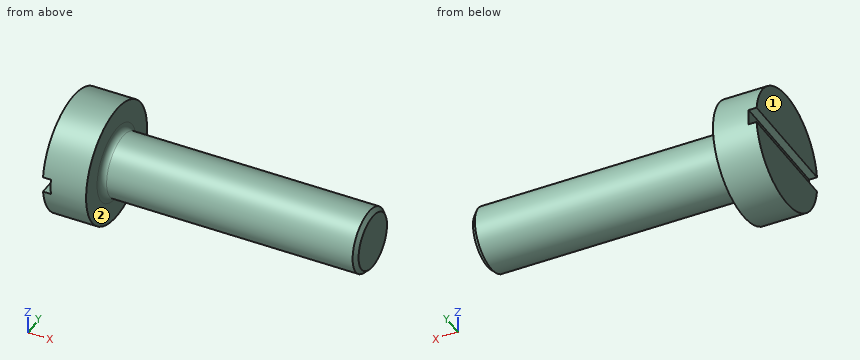
from build123d import *

# Parameters (mm, degrees)
SKETCH1_W           = 6.5
SKETCH1_H           = 0.8
CHAMFER1_SIZE       = 0.1
FILLET1_R           = 0.16
EXTRUDE1_DEPTH      = 8.890500618
EXTRUDE1_DEPTH_BACK = 8.890500618
SKETCH2_W           = 0.2
SKETCH2_H           = 0.2


with BuildPart() as part:
    # Sketch1 → Revolve1 (revolve)
    with BuildSketch(Plane.XY, mode=Mode.PRIVATE) as revolve1_sk:
        Polygon((0, 1.5), (0, 0), (1.1, 0), (1.1, 0.8), (1.1, 1.5), align=None)
        with Locations((4.35, 0.4)):
            Rectangle(SKETCH1_W, SKETCH1_H)
    revolve(revolve1_sk.sketch.rotate(Axis((0, 0, 0), (1, 0, 0)), 90), axis=Axis((0, 0, 0), (1, 0, 0)))

    # Chamfer1
    chamfer1_edges = [part.edges().sort_by_distance(p)[0] for p in [
        (7.6, 0, -0.8),
    ]]
    chamfer(chamfer1_edges, length=CHAMFER1_SIZE)

    # Fillet1
    fillet1_edges = [part.edges().sort_by_distance(p)[0] for p in [
        (1.1, 0, -0.8),
    ]]
    fillet(fillet1_edges, radius=FILLET1_R)

    # Sketch2 → Extrude1 (cut, two sides: drawn at the far end of the back side and taken through both)
    with BuildSketch(Plane(origin=(0, 0, 0), x_dir=(1, 0, 0), z_dir=(0, 1, 0)).offset(-EXTRUDE1_DEPTH_BACK)):
        with Locations((0.1, -0.1)):
            Rectangle(SKETCH2_W, SKETCH2_H)
        with Locations((0.1, 0.1)):
            Rectangle(SKETCH2_W, SKETCH2_H)
    extrude(amount=EXTRUDE1_DEPTH + EXTRUDE1_DEPTH_BACK, mode=Mode.SUBTRACT)


solid = part.part
Can you work these out from the model? Positions are in its coordinate system, mm. Face numbers are marked on the shaded views. A direction names the side the tool comes from. Coordinates: 2 decimals unless noted, no trailing zeros. Order: outer loops, then holes, each group sorted by start corner. A loop starts at its lowest first (then second) coordinate and runs counter-clockwise, first axis right, second up. Notation, with made-up numbers: (24.25, -23.75) - (32.25, -23.75) arc R25 ccw to (32.25, 0.25) - close; hole circle Ø3 at (-28.75, 27). An arc over 180 degrees is marked (long way). Answer as a JSON object with one key per item and string values. Group by question number.
Q1. On a 3-axis mill with a long thin cutter (end or side, diameter ignored), from which of +Z, -Z, +X, -X, +Y, -Y can I reach the whole of each face in a straight line? I mean the marked faces 1 and 2. Say none if no direction works.
Q2. Imagine slicing it at B-B (z = 0). Please give me the cut outline in (x, y), and give its area (3 significant figures).
Q3. Will this pin go through, and if not, where does the flat tip stop? P1, Ø1.5, axis at x = 1.5, z = 0.5, coming from the -Y side.
Q4. Imagine slicing it at A-A (y = 1.2). Please give me the cut outline in (x, z).
Q5. I need wall thicknesses on line 1 (X direction, y = -0.75, z = 1.15); line 2 (X direction, y = -1.35, z = 0); line 3 (Y direction, x = 7, z = -0.7). Which ranges of each line are inside material? Lowest first, please. Write a range as from..to.
Q6. Imagine slicing it at D-D (y = 0). Please give me the cut outline in (x, z), and give its area (3 significant figures).
Q7. Imagine slicing it at C-C (x = 1). Please give me the cut outline in (y, z), and give its area (3 significant figures).
Determined:
{
 "1": {"face 1": "+Z, -Z, -X, +Y, -Y", "face 2": "+X"},
 "2": {"outline": "(0.2, -1.5) - (1.1, -1.5) - (1.1, -0.96) arc R0.16 cw to (1.26, -0.8) - (7.5, -0.8) - (7.6, -0.7) - (7.6, 0.7) - (7.5, 0.8) - (1.26, 0.8) arc R0.16 cw to (1.1, 0.96) - (1.1, 1.5) - (0.2, 1.5) - close", "area": "13.1 mm2"},
 "3": {"P1": "stops at y = -1.5"},
 "4": {"outline": "(0, -0.9) - (1.1, -0.9) - (1.1, 0.9) - (0, 0.9) - (0, 0.2) - (0.2, 0.2) - (0.2, -0.2) - (0, -0.2) - close"},
 "5": {"line 1": "x = 0..1.1", "line 2": "x = 0.2..1.1", "line 3": "y = -0.39..0.39"},
 "6": {"outline": "(0, -1.5) - (1.1, -1.5) - (1.1, -0.96) arc R0.16 cw to (1.26, -0.8) - (7.5, -0.8) - (7.6, -0.7) - (7.6, 0.7) - (7.5, 0.8) - (1.26, 0.8) arc R0.16 cw to (1.1, 0.96) - (1.1, 1.5) - (0, 1.5) - (0, 0.2) - (0.2, 0.2) - (0.2, -0.2) - (0, -0.2) - close", "area": "13.6 mm2"},
 "7": {"outline": "circle Ø3 at (0, 0)", "area": "7.07 mm2"}
}
